For this review, take the finished solid that the model builds, in its own axes (mm). A direction names the side the tool comes from. Give positions to 0.01 mm unless a question says otherwise; leave off trailing zeros. Loops run counter-clockwise (first coordinate to the right, second up) from the corner with the lowest first, then second, coordinate; pieces in that order, holes last.
```python
from build123d import *

# Parameters (mm, degrees)
F1_DEPTH = 15


with BuildPart() as f1:
    # F0 (on Front) → F1 (new body)
    with BuildSketch(Plane.XZ):
        with BuildLine():
            Line((-562.4999962747, 150), (-619.9999962747, 150))
            Line((-619.9999962747, 150), (-619.9999962747, -50))
            ThreePointArc((-619.9999962747, -50), (-590.7106743934, -120.7106781187), (-519.9999962747, -150))
            Line((-519.9999962747, -150), (-499.9999962747, -150))
            Line((-499.9999962747, -150), (-499.9999962747, 0))
            Line((-499.9999962747, 0), (-484.9999962747, 0))
            Line((-484.9999962747, 0), (-484.9999962747, -150))
            ThreePointArc((-484.9999962747, -150), (-414.2893181561, -120.7106781187), (-384.9999962747, -50))
            add(Edge.make_bspline(
                [(-384.9999962747, -50), (-382.0572340786, -33.017525677), (-371.5647129158, 27.5340783447), (-1.601e-07, 110.9436321668), (371.5647207222, 27.5340787999), (382.0572416235, -33.0175256718), (385.0000037253, -50)],
                knots=[0, 0, 0, 0, 0.1402314153, 0.4999999982, 0.8597685847, 1, 1, 1, 1], degree=3))
            ThreePointArc((385.0000037253, -50), (414.2893256066, -120.7106781187), (485.0000037253, -150))
            Line((485.0000037253, -150), (485.0000037253, 0))
            Line((485.0000037253, 0), (500.0000037253, 0))
            Line((500.0000037253, 0), (500.0000037253, -150))
            Line((500.0000037253, -150), (520.0000037253, -150))
            ThreePointArc((520.0000037253, -150), (590.7106818439, -120.7106781187), (620.0000037253, -50))
            Line((620.0000037253, -50), (620.0000037253, 150))
            Line((620.0000037253, 150), (562.5000037253, 150))
            Line((562.5000037253, 150), (562.5000037253, 165))
            Line((562.5000037253, 165), (422.5000037253, 165))
            Line((422.5000037253, 165), (422.5000037253, 150))
            Line((422.5000037253, 150), (-422.4999962747, 150))
            Line((-422.4999962747, 150), (-422.4999962747, 165))
            Line((-422.4999962747, 165), (-562.4999962747, 165))
            Line((-562.4999962747, 165), (-562.4999962747, 150))
        make_face()
    extrude(amount=F1_DEPTH)


solid = f1.part
```
Item 1: Tool access review of faces 4 (the flat face through (-9, 0, 80)), 5 (the cylindrical face through (413.516, -7.395, -119.929)): name each direction out of +Z, -Z, +X, -X, +Y, -Y from which nothing blocks a thin tool from reaching the whole face with its end or side.
Answer:
face 4: +Z, -Z, +X, -X, +Y
face 5: -Z, +Y, -Y
Item 2: Clearance check with flat-ended pins moving along their axes: pin 1 Ø12 at (x, z) = (172, 54.5) entering from -Y; pin 2 Ø7.5 at (x, y) = (583.5, -4.5) entering from +Z; pin 3 Ø7.5 at (y, z) = (-8.5, 155) entering from +X; pin 4 Ø4.5 at (y, z) = (-7, 159.5) entering from -X. State where each tip first meets the part, or that it passes through.
Answer:
pin 1: passes through
pin 2: stops at z = 150
pin 3: stops at x = 562.5
pin 4: stops at x = -562.5
Item 3: Take a section at A-A on z = -94. Give the boundary of the cut face in (x, y), and give its area (3 significant figures).
Answer:
outline: (-609.8, -15) - (-500, -15) - (-500, 0) - (-609.8, 0) - close; (-485, -15) - (-395.2, -15) - (-395.2, 0) - (-485, 0) - close; (395.2, -15) - (485, -15) - (485, 0) - (395.2, 0) - close; (500, -15) - (609.8, -15) - (609.8, 0) - (500, 0) - close
area: 5,990 mm2
Item 4: The part is to be moulded in two halves that separate along X. For faces 1 (the cylindrical face through (589.929, -7.395, -121.484)), 2 (the cylindrical face through (-415.071, -7.395, -121.484)), 3 (the flat face through (-9, -15, 80)), say which applies: released by +X, released by -X, zero draft, split by the parting line, or undercut.
Answer:
face 1: released by +X
face 2: undercut
face 3: zero draft
Item 5: For L1, parallel to X at y = -8.5, z = -131; L2, parallel to X at y = -11.5, z = -31; L3, parallel to Z at x = 522.5, y = -4.5, list the stretches that pass through material, from the lowest coordinate up.
Answer:
L1: x = -578.64 to -500, -485 to -426.36, 426.36 to 485, 500 to 578.64
L2: x = -620 to -500, -485 to -380.85, 380.85 to 485, 500 to 620
L3: z = -149.97 to 165
